Input: part model. Units: mm. Frame: model coordinates. Face numbers are marked on the shaded views. A direction names the side the tool comes from. Give positions to 0.01 mm unless a question says otherwise; leave off trailing zeros. Loops run counter-clockwise (first coordinate to the right, second up) from the corner with the lowest first, then second, coordinate; pieces in that order, holes last. Notation, with made-up numbers: (62, 0.5) - (72, 0.5) arc R33 cw to (72, 33.5) - close; hole circle Ø1 at (45, -38). An arc over 180 degrees is marked (long way). Answer as a JSON object with one key per item and string values.
from build123d import *

# Parameters (mm, degrees)
EXTRUDE_1_DEPTH          = 2
EXTRUDE_2_DEPTH          = 12
SKETCH_5_R               = 3
CUT_EXTRUDE_1_DEPTH      = 15
SKETCH_8_W               = 16.6
SKETCH_8_H               = 9
CUT_EXTRUDE_3_DEPTH      = 7
CUT_EXTRUDE_5_DEPTH      = 1
CUT_EXTRUDE_5_DEPTH_BACK = 15
SKETCH_11_W              = 5
SKETCH_11_H              = 77
CUT_EXTRUDE_6_DEPTH      = 2


with BuildPart() as part:
    # 草图1 → 凸台-拉伸1 (new body)
    with BuildSketch(Plane.XY):
        with BuildLine():
            Line((0, 0), (8, 0))
            Line((8, 0), (8, 77))
            Line((8, 77), (0, 77))
            ThreePointArc((0, 77), (-5, 82), (0, 87))
            Line((0, 87), (79, 87))
            ThreePointArc((79, 87), (84, 82), (79, 77))
            Line((79, 77), (71, 77))
            Line((71, 77), (71, 0))
            Line((71, 0), (79, 0))
            ThreePointArc((79, 0), (84, -5), (79, -10))
            Line((79, -10), (71, -10))
            Line((71, -10), (8, -10))
            Line((8, -10), (0, -10))
            ThreePointArc((0, -10), (-5, -5), (0, 0))
        make_face()
    extrude(amount=EXTRUDE_1_DEPTH)

    # 草图4 → 凸台-拉伸2 (add)
    with BuildSketch(Plane(origin=(0, 0, 0), x_dir=(-1, 0, 0), z_dir=(0, 0, -1))):
        with BuildLine():
            Line((-11.3, 81), (-11.3, -10))
            Line((-11.3, -10), (0, -10))
            ThreePointArc((0, -10), (5, -5), (0, 0))
            Line((0, 0), (-8, 0))
            Line((-8, 0), (-8, 77))
            Line((-8, 77), (0, 77))
            ThreePointArc((0, 77), (5, 82), (0, 87))
            Line((0, 87), (-79, 87))
            ThreePointArc((-79, 87), (-84, 82), (-79, 77))
            Line((-79, 77), (-71, 77))
            Line((-71, 77), (-71, 0))
            Line((-71, 0), (-79, 0))
            ThreePointArc((-79, 0), (-84, -5), (-79, -10))
            Line((-79, -10), (-67.7, -10))
            Line((-67.7, -10), (-67.7, 81))
            Line((-67.7, 81), (-11.3, 81))
        make_face()
    extrude(amount=EXTRUDE_2_DEPTH)

    # 草图5 → 切除-拉伸1 (cut, through all)
    with BuildSketch(Plane.XY.offset(2)):
        with Locations((79, 82)):
            Circle(SKETCH_5_R)
        with Locations((0, 82)):
            Circle(SKETCH_5_R)
        with Locations((79, -5)):
            Circle(SKETCH_5_R)
        with Locations((0, -5)):
            Circle(SKETCH_5_R)
    extrude(amount=-CUT_EXTRUDE_1_DEPTH, mode=Mode.SUBTRACT)

    # 草图8 → 切除-拉伸3 (cut, through all)
    with BuildSketch(Plane.XZ.offset(-81)):
        with Locations((22.8, -7.5)):
            Rectangle(SKETCH_8_W, SKETCH_8_H)
    extrude(amount=-CUT_EXTRUDE_3_DEPTH, mode=Mode.SUBTRACT)

    # 草图10 → 切除-拉伸5 (cut, two sides)
    with BuildSketch(Plane(origin=(0, 0, -12), x_dir=(-1, 0, 0), z_dir=(0, 0, -1))) as cut_extrude_5_sk:
        Polygon((-290.643675891, 234.868702326), (-75.001818332, 87), (-68.001818332, 82.2), (-11, 82.2), (-4, 87), (211.641857559, 234.868702326), (211.641857559, 757.808713643), (-290.643675891, 757.808713643), align=None)
    extrude(amount=CUT_EXTRUDE_5_DEPTH, mode=Mode.SUBTRACT)
    extrude(cut_extrude_5_sk.sketch, amount=-CUT_EXTRUDE_5_DEPTH_BACK, mode=Mode.SUBTRACT)

    # 草图11 → 切除-拉伸6 (cut)
    with BuildSketch(Plane.XY.offset(2)):
        with Locations((14.5, 38.5)):
            Rectangle(SKETCH_11_W, SKETCH_11_H)
        with Locations((24.5, 38.5)):
            Rectangle(SKETCH_11_W, SKETCH_11_H)
        with Locations((34.5, 38.5)):
            Rectangle(SKETCH_11_W, SKETCH_11_H)
        with Locations((44.5, 38.5)):
            Rectangle(SKETCH_11_W, SKETCH_11_H)
        with Locations((54.5, 38.5)):
            Rectangle(SKETCH_11_W, SKETCH_11_H)
        with Locations((64.5, 38.5)):
            Rectangle(SKETCH_11_W, SKETCH_11_H)
    extrude(amount=-CUT_EXTRUDE_6_DEPTH, mode=Mode.SUBTRACT)


solid = part.part
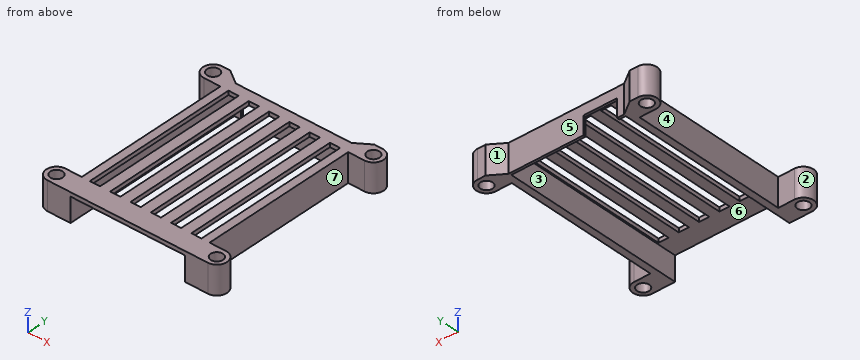
Item 1: Cut plane A-A (z = -5.25). Return loops of the section in (x, y), then the cut area to 3 significant figures.
Geometry check:
{"outline": "(0, -10) - (11.3, -10) - (11.3, 81) - (14.5, 81) - (14.5, 82.2) - (11, 82.2) - (4, 87) - (0, 87) arc R5 ccw to (0, 77) - (8, 77) - (8, 0) - (0, 0) arc R5 ccw to start; (31.1, 81) - (67.7, 81) - (67.7, -10) - (79, -10) arc R5 ccw to (79, 0) - (71, 0) - (71, 77) - (79, 77) arc R5 ccw to (79, 87) - (75, 87) - (68, 82.2) - (31.1, 82.2) - close; hole circle Ø6 at (0, -5); hole circle Ø6 at (0, 82); hole circle Ø6 at (79, -5); hole circle Ø6 at (79, 82)", "area": "1,020 mm2"}
Item 2: Cut plane B-B (x = 44). Return loops of the section in (y, z).
Geometry check:
{"outline": "(-10, 0) - (0, 0) - (0, 2) - (-10, 2) - close; (77, 0) - (81, 0) - (81, -12) - (82.2, -12) - (82.2, 2) - (77, 2) - close"}
Item 3: Contact query for flat-ended pins moving along their axis: P1, Ø6, axis at y = 44, z = -5, coming from the -X side; P2, Ø1, axis at y = 20, z = 1, coming from the +X side; P3, Ø1.5, axis at x = 42, z = -5.5, coming from the +Y side. Output: stop coordinate, or through.
Geometry check:
{"P1": "stops at x = 8", "P2": "stops at x = 71", "P3": "stops at y = 82.2"}
Item 4: Cut plane C-C (y = 70). Give the number of separate pieces and of enclosed holes in the cut face, then the cut area to 3 significant figures.
Geometry check:
{"separate pieces": "7", "enclosed holes": "0", "area": "145 mm2"}
Item 5: Access query for the marked faces 5, 6 and 7. Directions: +Z, -Z, +X, -X, +Y, -Y. A direction counts if a zero-diameter tool reaches every point of the face in a straight line with its end or side. Return the directions, or none.
Geometry check:
{"face 5": "+Z, -Z, +Y", "face 6": "-Z, -Y", "face 7": "+Z, -Z, +X"}
Item 6: Cut plane D-D (y = -5). Return loops of the section in (x, z), then the cut area to 3 significant figures.
Geometry check:
{"outline": "(-5, -12) - (-3, -12) - (-3, 2) - (-5, 2) - close; (3, -12) - (11.3, -12) - (11.3, 0) - (67.7, 0) - (67.7, -12) - (76, -12) - (76, 2) - (3, 2) - close; (82, -12) - (84, -12) - (84, 2) - (82, 2) - close", "area": "401 mm2"}
Item 7: Material intervals for line 1 (Y direction, x = 79, z = -1.25); line 2 (X direction, y = 71.5, z = -3.5); line 3 (Z direction, x = 18, y = 58.5), sorted ascending. Write a range as [from, to].
Geometry check:
{"line 1": "y = [-10, -8], [-2, 0], [77, 79], [85, 87]", "line 2": "x = [8, 11.3], [67.7, 71]", "line 3": "z = [0, 2]"}
Item 8: Mould query, pull axis Y, two halves, no side actions, for the marked faces 1, 2, 3 and 4. Classes: released by +Y, released by -Y, zero draft, split by the parting line, or undercut.
Geometry check:
{"face 1": "released by +Y", "face 2": "undercut", "face 3": "zero draft", "face 4": "undercut"}
